Autodesk Fusion 360 part; units mm, degrees
sketch "Sketch1" plane through (0, 0, 0) normal (0, 1, 0) x (1, 0, 0)
  line L0 (0, 0) -> (18.5729, 0) construction
  line L1 (18.5729, 0) -> (18.5729, -151.264) construction
  line L2 (18.5729, -151.264) -> (0, -151.264) construction
  line L3 (0, -151.264) -> (0, 0) construction
  line L4 (0, 0) -> (18.5729, -151.264) construction
  line L5 (0, 0) -> (43.3367, -352.9494) construction
  line L6 (-12.7, 12.7) -> (63.5, 12.7)
  line L7 (63.5, 12.7) -> (63.5, -368.3)
  line L8 (63.5, -368.3) -> (-12.7, -368.3)
  line L9 (-12.7, -368.3) -> (-12.7, 12.7)
  circle A0 centre (0, 0) radius 5
  circle A1 centre (18.5729, -151.264) radius 5
  circle A2 centre (43.3367, -352.9494) radius 4.7625
  line L10 (63.5, -368.3) -> (50.8, -368.3)
  line L11 (50.8, -368.3) -> (50.8, -337.82)
  line L12 (50.8, -337.82) -> (63.5, -337.82)
  line L13 (63.5, -337.82) -> (63.5, -368.3)
  line L14 (50.8, -353.06) -> (63.5, -353.06)
  dimension "d7" = 18.5729
  dimension "d8" = 151.264
  dimension "d9" = 355.6
  dimension "d10" = 381
  dimension "d11" = 76.2
  dimension "d13" = 12.7
  dimension "d14" = 12.7
  dimension "d15" = 10
  dimension "d16" = 10
  dimension "d19" = 9.525
  dimension "d22" = 30.48
  dimension "d23" = 12.7
extrude "Extrude1" add sketch "Sketch1" along normal blind 5.08 contours L6 L7 L8 L9 L11 L12 | L7 L11 L12 L13 L14 | L7 L8 L10 L11 L13 L14 | A2
extrude "Extrude3" add sketch "Sketch1" against normal blind 170.18 contours L7 L11 L12 L13 L14 | L7 L8 L10 L11 L13 L14
sketch "Sketch2" plane through (50.8, 0, 0) normal (-1, 0, 0) x (0, -1, 0)
  line L0 (0, 368.3) -> (0, 337.82)
  line L1 (0, 337.82) -> (170.18, 337.82)
  line L2 (170.18, 337.82) -> (170.18, 368.3)
  line L3 (170.18, 368.3) -> (0, 368.3)
  line L4 (85.09, 337.82) -> (85.09, 368.3)
  line L5 (170.18, 353.06) -> (0, 353.06)
  line L6 (59.69, 348.2975) -> (110.49, 348.2975) construction
  line L7 (110.49, 348.2975) -> (110.49, 357.8225) construction
  line L8 (110.49, 357.8225) -> (59.69, 357.8225) construction
  line L9 (59.69, 357.8225) -> (59.69, 348.2975) construction
  line L10 (59.69, 353.06) -> (110.49, 353.06)
  line L11 (85.09, 357.8225) -> (85.09, 348.2975)
  line L12 (110.49, 368.3) -> (115.57, 368.3)
  line L13 (115.57, 368.3) -> (115.57, 337.82)
  line L14 (115.57, 337.82) -> (110.49, 337.82)
  line L15 (110.49, 337.82) -> (110.49, 368.3)
  line L16 (54.61, 368.3) -> (54.61, 337.82)
  line L17 (59.69, 337.82) -> (59.69, 368.3)
  line L18 (59.69, 368.3) -> (54.61, 368.3)
  line L19 (54.61, 337.82) -> (59.69, 337.82)
  dimension "d26" = 9.525
  dimension "d27" = 50.8
  dimension "d28" = 30.48
  dimension "d29" = 85.09
  dimension "d30" = 5.08
  dimension "d31" = 5.08
  dimension "d32" = 30.48
extrude "Extrude4" add sketch "Sketch2" along normal blind 34.925 contours L3 L5 L16 L17 L18 | L1 L5 L16 L17 L19 | L3 L5 L12 L13 L15 | L1 L5 L13 L14 L15
hole "Hole1" at (33.3375, -59.69, 353.06) direction (0, 1, 0) diameter 9.525 depth 10.16 tip angle 118
hole "Hole2" at (33.3375, -115.57, 353.06) direction (0, 1, 0) diameter 9.525 depth 10.16 tip angle 118
sketch "Sketch3" plane through (0, -170.18, 0) normal (0, -1, 0) x (1, 0, 0)
  line L0 (50.8, 337.82) -> (63.5, 337.82)
  line L1 (63.5, 337.82) -> (63.5, 368.3)
  line L2 (63.5, 368.3) -> (50.8, 368.3)
  line L3 (50.8, 368.3) -> (50.8, 337.82)
  line L4 (63.5, 368.3) -> (-12.7, 368.3)
  line L5 (-12.7, 368.3) -> (-12.7, -12.7)
  line L6 (-12.7, -12.7) -> (63.5, -12.7)
  line L7 (63.5, -12.7) -> (63.5, 368.3)
  line L8 (0, 0) -> (18.5674, 0) construction
  line L9 (18.5674, 0) -> (18.5674, 151.257) construction
  line L10 (18.5674, 151.257) -> (0, 151.257) construction
  line L11 (0, 151.257) -> (0, 0) construction
  circle A0 centre (0, 0) radius 5
  line L12 (0, 0) -> (18.5674, 151.257) construction
  line L13 (0, 0) -> (43.3261, 352.9507) construction
  circle A1 centre (43.3261, 352.9507) radius 4.7625
  circle A2 centre (18.5674, 151.257) radius 5
  dimension "d41" = 381
  dimension "d42" = 76.2
  dimension "d43" = 151.257
  dimension "d44" = 18.5674
  dimension "d45" = 10
  dimension "d46" = 355.6
  dimension "d47" = 9.525
  dimension "d48" = 10
extrude "Extrude5" add 1 faces at (23.1881, 5.08, 297.6201) along direction (0, 1, 0) blind 1.27
extrude "Extrude6" add 1 faces at (20.1128, -54.61, 353.1786) along direction (0, 1, 0) blind 1.27
extrude "Extrude7" add 1 faces at (20.1128, -115.57, 353.1786) along direction (0, -1, 0) blind 1.27
extrude "Extrude8" add sketch "Sketch3" along normal blind 6.35 contours L0 L1 L2 L3 L4 L7 | L0 L3 L4 L5 L6 L7 | A1
equation "d19 = ( 3 / 8 ) * 1 in"
equation "d26 = ( 3 / 8 ) * 1 in"
Model file for the job. Use its own axes, mm. A direction names the side the tool comes from. Coordinates: 2 decimals unless noted, no trailing zeros. Loops run counter-clockwise (first coordinate to the right, second up) from the corner with the lowest first, then second, coordinate; pieces in that order, holes last. Notation, with made-up numbers: (-36, 28.25) -> (3, 28.25) arc R33 ccw to (3, 56.25) -> close; hole circle Ø1 at (86, -25.5). An arc over 180 degrees is marked (long way). Answer as a JSON object with one key per item and string values.
Q1. Flat gauge pins, fed straight in: P1, Ø3, axis at y = -112.5, z = 348, coming from the -X side (3 decimals); P2, Ø9, axis at y = -81, z = 355, coming from the -X side; P3, Ø9, axis at x = 18.57, z = 151.26, coming from the +Y side. Where does each tip first touch, or does it go through?
Report:
{"P1": "stops at x = 15.875", "P2": "stops at x = 50.8", "P3": "passes through"}
Q2. Cut at A-A (z = 0). List the corners of the cut face in (x, y), and give its area (3 significant figures).
Report:
{"outline": "(-12.7, -176.53) -> (-5, -176.53) -> (-5, -170.18) -> (-12.7, -170.18) -> close; (-12.7, 0) -> (-5, 0) -> (-5, 6.35) -> (-12.7, 6.35) -> close; (5, -176.53) -> (63.5, -176.53) -> (63.5, -170.18) -> (5, -170.18) -> close; (5, 0) -> (63.5, 0) -> (63.5, 6.35) -> (5, 6.35) -> close", "area": "841 mm2"}
Q3. Pull direction Y, two halves, no side cores. Call faces 6 (the flat face through (25, 6.35, 175)), 7 (the cylindrical face through (-1.08, 3.13, -4.88)), 8 (the flat face through (30, -116.84, 357)): released by +Y, released by -Y, zero draft, split by the parting line, or undercut.
Report:
{"face 6": "released by +Y", "face 7": "zero draft", "face 8": "undercut"}
Q4. Cut at C-C (z = 353.06). List the corners of the cut face in (x, y) (3 decimals).
Report:
{"outline": "(-12.7, -176.53) -> (63.5, -176.53) -> (63.5, 6.35) -> (-12.7, 6.35) -> (-12.7, 0) -> (50.8, 0) -> (50.8, -53.34) -> (38.1, -53.34) -> (38.1, -59.69) -> (50.8, -59.69) -> (50.8, -110.49) -> (38.1, -110.49) -> (38.1, -116.84) -> (50.8, -116.84) -> (50.8, -170.18) -> (-12.7, -170.18) -> close; (15.875, -116.84) -> (28.575, -116.84) -> (28.575, -110.49) -> (15.875, -110.49) -> close; (15.875, -59.69) -> (28.575, -59.69) -> (28.575, -53.34) -> (15.875, -53.34) -> close"}
Q5. 3-axis set-ups, long thin cutter, end or side, ignore diameter. For faces 1 (the flat face through (51, -78, 368.3)), 2 (the cylindrical face through (33.547, -56.559, 357.818)), 3 (the flat face through (54, -85, 337.82)), 4 (the cylindrical face through (-1.08, -173.31, 4.88)), 5 (the flat face through (30, -53.34, 357)): which of +Z, -Z, +X, -X, +Y, -Y reach the whole face in a straight line?
Report:
{"face 1": "+Z, +X, -X, +Y, -Y", "face 2": "none", "face 3": "-Z, +X, -X", "face 4": "+Y, -Y", "face 5": "+Z, -Z, -X"}
Q6. Cut at D-D (z = 175). List the corners of the cut face in (x, y).
Report:
{"outline": "(-12.7, -176.53) -> (63.5, -176.53) -> (63.5, -170.18) -> (-12.7, -170.18) -> close; (-12.7, 0) -> (63.5, 0) -> (63.5, 6.35) -> (-12.7, 6.35) -> close"}
Q7. Probe probe 1 along Y at (x, z) = (9, 315); probe 2 along Z at (x, y) = (0, 3); probe 3 along X at (y, z) = (1, 0). List the from-to ranges inside material, lowest first.
Report:
{"probe 1": "y = -176.53 to -170.18, 0 to 6.35", "probe 2": "z = -12.7 to -5, 5 to 368.3", "probe 3": "x = -12.7 to -5, 5 to 63.5"}
Q8. Cut at B-B (x = 0). List the corners of the cut face in (y, z), and give its area (3 significant figures).
Report:
{"outline": "(-176.53, -12.7) -> (-170.18, -12.7) -> (-170.18, -5) -> (-176.53, -5) -> close; (-176.53, 5) -> (-170.18, 5) -> (-170.18, 368.3) -> (-176.53, 368.3) -> close; (0, -12.7) -> (6.35, -12.7) -> (6.35, -5) -> (0, -5) -> close; (0, 5) -> (6.35, 5) -> (6.35, 368.3) -> (0, 368.3) -> close", "area": "4,710 mm2"}
